Check sheet for the modelled part. Datum: model origin and axes. Units: mm. A direction names the side the tool comes from. Round coordinates to 2 decimals unless told otherwise and drop trailing zeros. Write each loop counter-clockwise with the first axis right and the second up, starting at its lowest first coordinate (ties: lowest second). Pieces come first, ordered by that corner, then holes.
Autodesk Inventor part; units mm, degrees
ref_plane "YZ Plane" through (0, 0, 0) normal (1, 0, 0) x (0, 1, 0)
ref_plane "XZ Plane" through (0, 0, 0) normal (0, 1, 0) x (-1, 0, 0)
ref_plane "XY Plane" through (0, 0, 0) normal (0, 0, 1) x (1, 0, 0)
sketch "Esboço1" plane through (0, 0, 0) normal (0, 1, 0) x (-1, 0, 0)
  line L0 (-70, 60) -> (70, 60)
  line L1 (70, 60) -> (70, -60)
  line L2 (70, -60) -> (-70, -60)
  line L3 (-70, -60) -> (-70, 60)
  line L4 (-70, 60) -> (70, -60) construction
  line L5 (70, 60) -> (-70, -60) construction
  point P0 (0, 0)
  dimension "d0" = 140
  dimension "d1" = 120
extrude "Extrusão1" add sketch "Esboço1" along normal blind 1.6
sketch "Esboço2" plane through (0, 1.6, 0) normal (0, 1, 0) x (1, 0, 0)
  line L0 (-94.6357, 0) -> (83.6022, 0)
  line L1 (-70, -37) -> (-52, -37)
  line L2 (-52, 37) -> (-70, 37)
  line L3 (-70, 37) -> (-70, -37)
  line L4 (-70, -37) -> (-52, 37) construction
  line L5 (-52, -37) -> (-70, 37) construction
  line L6 (-70, 60) -> (-70, -60)
  line L7 (-70, 0) -> (-70, 0)
  line L8 (-70, 0) -> (-25, 0)
  circle A0 centre (-25, 0) radius 12.5
  line L9 (-70, -60) -> (70, -60)
  line L10 (-20, -60) -> (-50, -60)
  line L11 (-20, -60) -> (10, -60)
  line L12 (70, 60) -> (-70, 60)
  line L13 (-55, -60) -> (5, -60)
  line L14 (5, -60) -> (5, -45)
  line L15 (-55, -45) -> (-55, -60)
  line L16 (-52, 0) -> (-70, 0)
  line L17 (-56, 25) -> (-48, 25)
  line L18 (-48, 25) -> (-48, -25)
  line L19 (-48, -25) -> (-56, -25)
  line L20 (-56, -25) -> (-56, 25)
  line L21 (-56, 25) -> (-48, -25) construction
  line L22 (-48, 25) -> (-56, -25) construction
  line L23 (-55, 60) -> (5, 60)
  line L24 (5, 60) -> (5, 45)
  line L25 (-55, 45) -> (-55, 60)
  line L26 (-25, 76.0053) -> (-25, -77.5323)
  line L27 (-35, -45) -> (-35, -37)
  line L28 (-35, -37) -> (-15, -37)
  line L29 (-15, -37) -> (-15, -45)
  line L30 (5, -45) -> (-15, -45)
  line L31 (-35, -45) -> (-55, -45)
  line L32 (-35, 45) -> (-35, 37)
  line L33 (-35, 37) -> (-15, 37)
  line L34 (-15, 37) -> (-15, 45)
  line L35 (5, 45) -> (-15, 45)
  line L36 (-35, 45) -> (-55, 45)
  line L37 (-55, -60) -> (5, -45) construction
  line L38 (5, -60) -> (-55, -45) construction
  line L39 (-35, 45) -> (-15, 37) construction
  line L40 (-15, 45) -> (-35, 37) construction
  point P0 (0, 0)
  point P1 (-61, 0)
  point P2 (-25, 41)
  dimension "d4" = 18
  dimension "d5" = 74
  dimension "d6" = 0
  dimension "d7" = 45
  dimension "d8" = 25
  dimension "d28" = 15
  dimension "d30" = 18
  dimension "d31" = 8
  dimension "d32" = 50
  dimension "d35" = 15
  dimension "d36" = 20
  dimension "d38" = 8
  dimension "d40" = 20
  dimension "d41" = 8
  dimension "d42" = 60
  dimension "d43" = 60
extrude "Extrusão4" cut sketch "Esboço2" against normal through all contours L26 A0 L0 | L26 A0 L0 | L0 A0 L26 | L0 A0 L26 | L18 L19 L20 L0 | L0 L20 L17 L18
sketch "Esboço3" plane through (0, 1.6, 0) normal (0, 1, 0) x (1, 0, 0)
  line L0 (44.5, -40) -> (30, -40) construction
  line L1 (30, -40) -> (30, -72.5) construction
  line L2 (30, -72.5) -> (44.5, -72.5) construction
  line L3 (44.5, -72.5) -> (44.5, -40) construction
  line L4 (30, 40) -> (44.5, 40) construction
  line L5 (44.5, 40) -> (44.5, 72.5) construction
  line L6 (44.5, 72.5) -> (30, 72.5) construction
  line L7 (30, 72.5) -> (30, 40) construction
  line L8 (37.25, -40) -> (37.25, -47.2) construction
  circle A0 centre (37.25, -47.2) radius 1.5
  line L9 (37.25, 40) -> (37.25, 47.2) construction
  circle A1 centre (37.25, 47.2) radius 1.5
  line L10 (-70, 60) -> (-70, -60)
  line L11 (52, 14) -> (49.5, 14) construction
  line L12 (49.5, 14) -> (49.5, -14) construction
  line L13 (49.5, -14) -> (52, -14) construction
  line L14 (52, -14) -> (52, 14) construction
  line L15 (52, 14) -> (49.5, -14) construction
  line L16 (49.5, 14) -> (52, -14) construction
  line L17 (54, 16) -> (47.5, 16)
  line L18 (47.5, 16) -> (47.5, -16) construction
  line L19 (47.5, -16) -> (54, -16) construction
  line L20 (54, -16) -> (54, 16)
  line L21 (70, -60) -> (70, 60)
  line L22 (5, -54.0532) -> (28, -36.1915)
  line L23 (28, -36.1915) -> (28, -58)
  line L24 (44.5, -69.5) -> (44.5446, -69.5)
  line L25 (46.5, -58) -> (46.5, -38)
  line L26 (46.5, -38) -> (46.5, -36.8245)
  line L27 (46.5, -58) -> (28, -58)
  line L28 (-70, -60) -> (70, -60)
  line L29 (7, -60) -> (5, -60)
  line L30 (70, 60) -> (-70, 60)
  line L31 (70, 60) -> (7, 60)
  line L32 (5, 54.0532) -> (28, 36.1915)
  line L33 (28, 58) -> (28, 36.1915)
  line L34 (44.5446, 69.5) -> (44.5, 69.5)
  line L35 (46.5, 58) -> (28, 58)
  line L36 (46.5, 36.8245) -> (46.5, 58)
  line L37 (5, 54.0532) -> (5, 60)
  line L38 (5, -54.0532) -> (5, -60)
  line L39 (54, -16) -> (54, -31)
  line L40 (54, -31) -> (46.5, -36.8245)
  line L41 (54, 16) -> (54, 31)
  line L42 (54, 31) -> (46.5, 36.8245)
  point P0 (0, 0)
  dimension "d59" = 14.5
  dimension "d60" = 32.5
  dimension "d63" = 32.5
  dimension "d64" = 14.5
  dimension "d76" = 7.2
  dimension "d77" = 3
  dimension "d78" = 7.2
  dimension "d79" = 3
  dimension "d97" = 2.5
  dimension "d98" = 28
  dimension "d99" = 2
  dimension "d103" = 2
  dimension "d104" = 2
  dimension "d105" = 63
  dimension "d107" = 2
  dimension "d132" = 15
  dimension "d133" = 15
sketch "Esboço4" plane through (0, 1.6, 0) normal (0, 1, 0) x (1, 0, 0)
  line L0 (-70, 60) -> (-70, -60)
  line L1 (-70, 0) -> (-70, -100)
  line L2 (-70, -100) -> (180, -100)
  line L3 (180, -100) -> (180, 100)
  line L4 (180, 100) -> (-70, 100)
  line L5 (-70, 100) -> (-70, -100)
  line L6 (250, 0) -> (-150, 0)
  line L7 (-430, 10) -> (570, 10)
  line L8 (570, 10) -> (570, -10)
  line L9 (570, -10) -> (-430, -10)
  line L10 (-430, -10) -> (-430, 10)
  line L11 (70, -60) -> (70, 60)
  line L12 (-430, 10) -> (570, -10) construction
  line L13 (570, 10) -> (-430, -10) construction
  line L14 (27.5, -90) -> (47.5, -90)
  line L15 (47.5, -90) -> (47.5, -50)
  line L16 (47.5, -50) -> (27.5, -50)
  line L17 (27.5, -50) -> (27.5, -90)
  line L18 (27.5, -90) -> (47.5, -50) construction
  line L19 (47.5, -90) -> (27.5, -50) construction
  line L20 (70, 60) -> (-70, 60)
  line L21 (47.5, 90) -> (27.5, 90)
  line L22 (27.5, 90) -> (27.5, 50)
  line L23 (27.5, 50) -> (47.5, 50)
  line L24 (47.5, 50) -> (47.5, 90)
  line L25 (47.5, 90) -> (27.5, 50) construction
  line L26 (27.5, 90) -> (47.5, 50) construction
  line L27 (0, -100) -> (0, 100) construction
  point P0 (0, 0)
  point P1 (70, 0)
  point P2 (37.5, -70)
  point P3 (37.5, 70)
  dimension "d53" = 100
  dimension "d54" = 250
  dimension "d55" = 200
  dimension "d65" = 1000
  dimension "d66" = 20
  dimension "d68" = 20
  dimension "d69" = 40
  dimension "d70" = 20
  dimension "d71" = 40
  dimension "d72" = 40
  dimension "d73" = 40
  dimension "d80" = 37.5
  dimension "d81" = 37.5
extrude "Extrusão5" cut sketch "Esboço3" against normal through all contours A0 | A1
sketch "Esboço5" plane through (0, 1.6, 0) normal (0, 1, 0) x (1, 0, 0)
  line L0 (70, 60) -> (-70, 60)
  line L1 (-70, 60) -> (-55, 60)
  line L2 (-55, 60) -> (-55, 39)
  line L3 (-55, 39) -> (-70, 39)
  line L4 (-70, 39) -> (-70, 60)
  line L5 (-70, -60) -> (70, -60)
  line L6 (-70, -60) -> (-55, -60)
  line L7 (-55, -60) -> (-55, -39)
  line L8 (-55, -39) -> (-70, -39)
  line L9 (-70, -39) -> (-70, -60)
  line L10 (-70, 60) -> (-70, -60)
  line L11 (-55, 39) -> (-70, 39)
  line L12 (-70, 39) -> (-70, 60)
  line L13 (-70, 60) -> (-55, 60)
  line L14 (-55, 60) -> (-55, 39)
  line L15 (-55, -39) -> (-70, -39)
  line L16 (-70, -39) -> (-70, -60)
  line L17 (-70, -60) -> (-55, -60)
  line L18 (-55, -60) -> (-55, -39)
  point P0 (0, 0)
  dimension "d84" = 15
  dimension "d85" = 21
  dimension "d86" = 15
  dimension "d87" = 21
extrude "Extrusão6" cut sketch "Esboço5" against normal through all
fillet "Arredondamento1" radius 2 10 edges at (-70, 0.8, 39) (-55, 0.8, 39) (-55, 0.8, 60) (-56, 0.8, 25) (-48, 0.8, 25) (-56, 0.8, -25) (-48, 0.8, -25) (-70, 0.8, -39) (-55, 0.8, -39) (-55, 0.8, -60)
sketch "Esboço7" plane through (0, 1.6, 0) normal (0, 1, 0) x (1, 0, 0)
  line L0 (-3.4695, -17.196) -> (-3.4695, -2.1961) construction
  line L1 (-3.4695, -2.1961) -> (11.6526, -2.1961) construction
  line L2 (11.6526, -2.1961) -> (11.6526, -17.196) construction
  line L3 (11.6526, -17.196) -> (-3.4695, -17.196) construction
  point P0 (0, 0)
extrude "Extrusão10" cut sketch "Esboço3" against normal through all contours L30 L21 L28 L38 L22 L23 L27 L25 L26 L40 L39 L20 L41 L42 L36 L35 L33 L32 L37
fillet "Arredondamento4" radius 2 14 edges at (5, 0.8, 60) (5, 0.8, 54.0532) (28, 0.8, 36.1915) (28, 0.8, 58) (46.5, 0.8, 58) (46.5, 0.8, 36.8245) (54, 0.8, 31) (54, 0.8, -31) (46.5, 0.8, -36.8245) (46.5, 0.8, -58) (28, 0.8, -58) (28, 0.8, -36.1915) (5, 0.8, -54.0532) (5, 0.8, -60)
properties part number "PCB"
1. Sectioned sample at A-A, the plane z = -17. Enter the section's corners in (x, y), plus the area to 3 significant figures.
2. Sectioned sample at C-C, the plane z = 0. Enter the section's corners in (x, y).
3. Sectioned sample at D-D, the plane y = 1.05. Give the number of separate pieces and of enclosed holes in the cut face, plus the area to 3 significant figures.
4. Go/stop test with flat-tipped pins: pin 1 (0.5 mm diameter, centred on y = 1, z = 51.5, fed in from -X); pin 2 (0.8 mm diameter, centred on x = -63.5, y = 1, fed in from +Z); pin 3 (0.8 mm diameter, centred on x = -62, y = 1, fed in from -Z). Record where each tip stops, or that it passes through.
5. Sectioned sample at B-B, the plane x = -25. Enter the section's corners in (y, z).
6. Release check for a two-part mould opening along X. For faces 1 (the flat face through (-7, 1.6, 1)), 2 (the flat face through (50.29, 0.81, 33.88)), 3 (the cylindrical face through (36.14, 0.81, -48.21)), 4 (the cylindrical face through (-34.92, 0.811, 7.606)) record: released by +X, released by -X, zero draft, split by the parting line, or undercut.
7. Scan lines: line 1 along Z through (x, y) = (37.25, 0.65); line 2 along X through (y, z) = (0.5, 0); line 3 along X through (y, z) = (0.5, -47.2). Record each from-to range of solid material in increasing order.
8. Set-up check for faces 5 (the flat face through (-7, 0, 1)), 6 (the flat face through (15.14, 0.81, 46.18)), 7 (the flat face through (15.14, 0.81, -46.18)): record each of +Z, -Z, +X, -X, +Y, -Y from which the full face is reachable in a straight line by a thin tool's end or side.
Computed values:
1. outline: (-70, 0) - (-56, 0) - (-56, 1.6) - (-70, 1.6) - close; (-48, 0) - (54, 0) - (54, 1.6) - (-48, 1.6) - close
1. area: 186 mm2
2. outline: (-70, 0) - (-56, 0) - (-56, 1.6) - (-70, 1.6) - close; (-48, 0) - (-37.5, 0) - (-37.5, 1.6) - (-48, 1.6) - close; (-12.5, 0) - (54, 0) - (54, 1.6) - (-12.5, 1.6) - close
3. separate pieces: 1
3. enclosed holes: 4
3. area: 12,200 mm2
4. pin 1: stops at x = -55
4. pin 2: stops at z = 39
4. pin 3: stops at z = -39
5. outline: (0, -60) - (1.6, -60) - (1.6, -12.5) - (0, -12.5) - close; (0, 12.5) - (1.6, 12.5) - (1.6, 60) - (0, 60) - close
6. face 1: zero draft
6. face 2: released by +X
6. face 3: undercut
6. face 4: undercut
7. line 1: z = -58 to -48.7, -45.7 to 45.7, 48.7 to 58
7. line 2: x = -70 to -56, -48 to -37.5, -12.5 to 54
7. line 3: x = -55 to 13.82, 28 to 35.75, 38.75 to 46.5
8. face 5: +Z, -Z, +X, -X, -Y
8. face 6: +Z, +Y, -Y
8. face 7: -Z, +Y, -Y
